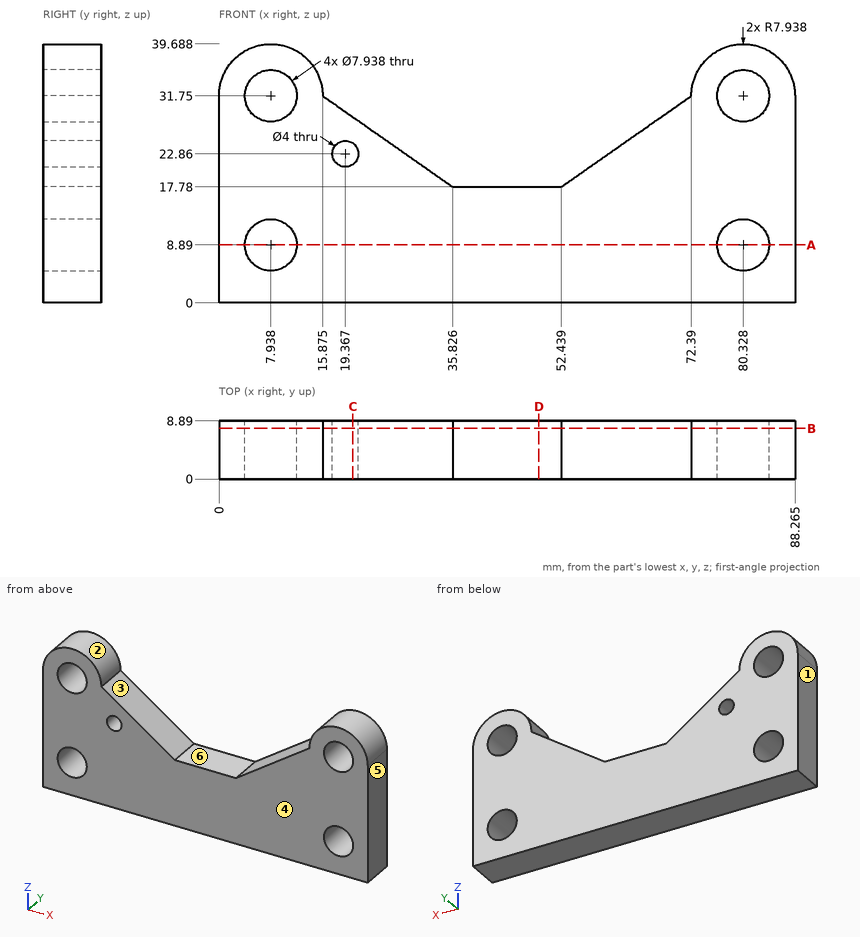
Answer from the drawing. Dimensions are ordinates in mm from the lowest x, y and z of the part. A direction names the side the tool comes from. Round coordinates to 2 decimals unless told otherwise and drop trailing zeros. Order: outer loops, then holes, each group sorted by start corner. A loop starts at its lowest first (then second) coordinate and runs counter-clockwise, first axis right, second up. Notation, with made-up numbers: (61, 57.5) -> (65, 57.5) arc R25 cw to (65, 94.5) -> close; hole circle Ø8 at (-32, -2). An arc over 180 degrees is marked (long way). Answer as CSV lines item,"result".
Q1. A cutting plane is placed at D-D on x = 49. Determine the outline of the cut face in (y, z), plus the area to 3 significant figures.
Computed values:
outline,"(0, 0) -> (8.89, 0) -> (8.89, 17.78) -> (0, 17.78) -> close"
area,"158 mm^2"
Q2. A cutting plane is placed at B-B on y = 7.75. Give the number of separate pieces and of enclosed holes in the cut face, plus the area to 3 significant figures.
Computed values:
separate pieces,"1"
enclosed holes,"5"
area,"2,280 mm^2"
Q3. A cutting plane is placed at C-C on x = 20.5. Determine the outline of the cut face in (y, z).
Computed values:
outline,"(0, 0) -> (8.89, 0) -> (8.89, 21.21) -> (0, 21.21) -> close; (0, 24.51) -> (8.89, 24.51) -> (8.89, 28.51) -> (0, 28.51) -> close"
Q4. Consider line 1 (X direction, y = 3.25, z = 31.75) (1 decimal); line 2 (X direction, y = 7, z = 8.89) (1 decimal); line 3 (X direction, y = 8.5, z = 23.5) (1 decimal). Determine where each line is inside the solid, lowest interval first. Write a range as from..to.
Computed values:
line 1,"x = 0..4, 11.9..15.9, 72.4..76.4, 84.3..88.3"
line 2,"x = 0..4, 11.9..76.4, 84.3..88.3"
line 3,"x = 0..17.5, 21.3..27.7, 60.6..88.3"
Q5. Which of the six approach directions +Z, -Z, +X, -X, +Y, -Y give full straight-line access (tool end or side, diameter ignored) to the marked faces 5 and 6?
Computed values:
face 5,"+Z, -Z, +X, +Y, -Y"
face 6,"+Z, +Y, -Y"
Q6. A cutting plane is placed at A-A on z = 8.89. Determine the outline of the cut face in (x, y) (1 decimal).
Computed values:
outline,"(0, 0) -> (4, 0) -> (4, 8.9) -> (0, 8.9) -> close; (11.9, 0) -> (76.4, 0) -> (76.4, 8.9) -> (11.9, 8.9) -> close; (84.3, 0) -> (88.3, 0) -> (88.3, 8.9) -> (84.3, 8.9) -> close"
Q7. For a pull along X with two mould halves and no side action, classify the marked faces 1, 2, 3 and 4 as +X half, -X half, draft (parallel to the pull), parting line (faces both ways), or undercut.
Computed values:
face 1,"-X half"
face 2,"undercut"
face 3,"undercut"
face 4,"draft"
